Read the model definition and answer for the solid it produces. Units are mm, in the model's axes. A direction names the side the tool comes from. Give positions to 0.01 mm unless a question says otherwise; leave off trailing zeros. Loops run counter-clockwise (first coordinate to the right, second up) from the corner with the lowest first, then second, coordinate; pieces in that order, holes last. Notation, with made-up numbers: (-20, -18.5) -> (-14, -18.5) arc R26 ccw to (-14, -3.5) -> close; hole circle Ø8 at (19, 26). An arc over 180 degrees is marked (long way). Return JSON: item names as keys, results as strings. Group by question number.
from build123d import *

# Parameters (mm, degrees)
SALIENTE_EXTRUIR1_DEPTH                     = 31.75
CROQUIS1_R                                  = 9.525
CROQUIS1_R_2                                = 25.4
SALIENTE_EXTRUIR1_2_DEPTH                   = 31.75
SALIENTE_EXTRUIR2_DEPTH                     = 82.55
SALIENTE_EXTRUIR3_REACH                     = 71.85
TALADRO1_D                                  = 25.4
REFRENTADO_PARA_TORNILLO_CON_CABEZA_2_COUNT = 2
REFRENTADO_PARA_TORNILLO_CON_CABEZA_2_PITCH = 56.896
REFRENTADO_PARA_TORNILLO_CON_CABEZA_3_COUNT = 2
REFRENTADO_PARA_TORNILLO_CON_CABEZA_3_PITCH = 110.426919924


with BuildPart() as part:
    # Croquis1 → Saliente-Extruir1 (new body)
    with BuildSketch(Plane.XY):
        with BuildLine():
            Line((50.8, 170.942), (12.7, 170.942))
            Line((12.7, 170.942), (12.7, 154.94))
            Line((12.7, 154.94), (-12.7, 154.94))
            Line((-12.7, 154.94), (-12.7, 170.942))
            Line((-12.7, 170.942), (-50.8, 170.942))
            ThreePointArc((-50.8, 170.942), (-55.290128061, 169.082128061), (-57.15, 164.592))
            Line((-57.15, 164.592), (-57.15, 101.092))
            ThreePointArc((-57.15, 101.092), (-55.290128061, 105.582128061), (-50.8, 107.442))
            Line((-50.8, 107.442), (50.8, 107.442))
            ThreePointArc((50.8, 107.442), (55.290128061, 105.582128061), (57.15, 101.092))
            Line((57.15, 101.092), (57.15, 164.592))
            ThreePointArc((57.15, 164.592), (55.290128061, 169.082128061), (50.8, 170.942))
        make_face()
    extrude(amount=SALIENTE_EXTRUIR1_DEPTH)



with BuildPart() as body_2:
    # Croquis1 → Saliente-Extruir1 2 (new body)
    with BuildSketch(Plane.XY):
        with BuildLine():
            Line((57.15, 0), (57.15, 75.692))
            ThreePointArc((57.15, 75.692), (55.290128061, 71.201871939), (50.8, 69.342))
            Line((50.8, 69.342), (-50.8, 69.342))
            ThreePointArc((-50.8, 69.342), (-55.290128061, 71.201871939), (-57.15, 75.692))
            Line((-57.15, 75.692), (-57.15, 0))
            ThreePointArc((-57.15, 0), (0, -57.15), (57.15, 0))
        make_face()
        with Locations((0, -41.402)):
            Circle(CROQUIS1_R, mode=Mode.SUBTRACT)
        Circle(CROQUIS1_R_2, mode=Mode.SUBTRACT)
    extrude(amount=SALIENTE_EXTRUIR1_2_DEPTH)


with BuildPart() as part_1:
    add(part.part)

    add(body_2.part)  # Saliente-Extruir2 merges body 2
    # Croquis1_3 → Saliente-Extruir2 (add)
    with BuildSketch(Plane.XY):
        with BuildLine():
            Line((57.15, 75.692), (57.15, 101.092))
            ThreePointArc((57.15, 101.092), (55.290128061, 105.582128061), (50.8, 107.442))
            Line((50.8, 107.442), (-50.8, 107.442))
            ThreePointArc((-50.8, 107.442), (-55.290128061, 105.582128061), (-57.15, 101.092))
            Line((-57.15, 101.092), (-57.15, 75.692))
            ThreePointArc((-57.15, 75.692), (-55.290128061, 71.201871939), (-50.8, 69.342))
            Line((-50.8, 69.342), (50.8, 69.342))
            ThreePointArc((50.8, 69.342), (55.290128061, 71.201871939), (57.15, 75.692))
        make_face()
    extrude(amount=SALIENTE_EXTRUIR2_DEPTH)

    # Croquis4 → Saliente-Extruir3 (add, up to next)
    with BuildSketch(Plane.ZY.offset(-12.7), mode=Mode.PRIVATE) as saliente_extruir3_sk1:
        Polygon((31.75, 154.94), (0, 170.942), (0, 154.94), align=None)
    saliente_extruir3_tool1 = extrude(saliente_extruir3_sk1.sketch, amount=SALIENTE_EXTRUIR3_REACH, mode=Mode.PRIVATE) - part_1.part
    add(saliente_extruir3_tool1.solids().sort_by_distance((12.7, 160.274, 10.583333))[0])

    # Taladro1 (through all)
    with Locations(Plane(origin=(0, 107.442, 0), x_dir=(1, 0, 0), z_dir=(0, 1, 0))):
        with Locations((0, -57.15)):
            Hole(TALADRO1_D / 2)

    # Croquis10 → Refrentado para tornillo con cabeza tron (revolve, cut)
    with BuildSketch(Plane(origin=(28.448, 135.89, 31.75), x_dir=(0, -1, 0), z_dir=(1, 0, 0))):
        Polygon((0, 0), (0, 31.75), (6.35, 31.75), (6.35, 8.350483939), (6.985, 7.62), (8.001, 7.62), (8.001, 0), align=None)
    refrentado_para_tornillo_con_cabeza_tron = revolve(axis=Axis((28.448, 135.89, 38.1), (0, 0, -1)), mode=Mode.SUBTRACT)

    # Refrentado para tornillo con cabeza  2: Refrentado para tornillo con cabeza tron ×2
    with Locations(*[(-i * REFRENTADO_PARA_TORNILLO_CON_CABEZA_2_PITCH, 0, 0) for i in range(1, REFRENTADO_PARA_TORNILLO_CON_CABEZA_2_COUNT)]):
        add(refrentado_para_tornillo_con_cabeza_tron, mode=Mode.SUBTRACT)

    # Refrentado para tornillo con cabeza  3: Refrentado para tornillo con cabeza tron ×2
    with Locations(*[Vector(-0.517536847, -0.855660921, 0) * (i * REFRENTADO_PARA_TORNILLO_CON_CABEZA_3_PITCH) for i in range(1, REFRENTADO_PARA_TORNILLO_CON_CABEZA_3_COUNT)]):
        add(refrentado_para_tornillo_con_cabeza_tron, mode=Mode.SUBTRACT)


solid = part_1.part
1. Flat-ended cylindrical pins translate along their axes: pin 1 Ø5 at (y, z) = (49, 34) entering from +X; pin 2 Ø16.5 at (x, y) = (-28.448, 135.89) entering from +Z; pin 3 Ø1.5 at (x, z) = (45, 65) entering from -Y; pin 4 Ø9.5 at (x, y) = (28.448, 135.89) entering from -Z. Find the tip coordinate at first contact, or state that the pin passes through.
2. Straight lines are drawn through the part: line 1 (X direction, y = 135.89, z = 27); line 2 (X direction, y = 135.89, z = 18.25); line 3 (Z direction, x = 0, y = 79). For each, find the intervals that lie inside material, in ascending order. Write a range as from..to.
3. Section A-A on y = 135.89 is taken. Determine the outline of the cut face in (x, z).
4. Determine the mould class of faces 4 (the cylindrical face through (-55.34, 71.25, 56.79)), 5 (the cylindrical face through (-24.584, 140.929, 11.864)), 6 (the cylindrical face through (55.34, 169.03, 15.65)), 7 (the flat face through (12, 25, 31.75)) for opening direction X: pulls with the +X half, pulls with the -X half, needs draft (parallel to the pull), parting line crosses it, or undercut.
5. Section C-C on x = 0 is taken. Determine the outline of the cut face in (y, z).
6. Which of the six approach directions +Z, -Z, +X, -X, +Y, -Y give full straight-line access (tool end or side, diameter ignored) to faces 1 (the cylindrical face through (28.096, 143.883, 27.993)), 2 (the cylindrical face through (55.24, 71.15, 56.79)), 3 (the flat face through (12, 107.442, 51))?
7. Section D-D on z = 75.5 is taken. Determine the outline of the cut face in (x, y), then the cut area to 3 significant figures.
8. Section B-B on z = 57.15 is taken. Determine the outline of the cut face in (x, y).
Completed:
{
 "1": {"pin 1": "stops at x = 57.15", "pin 2": "stops at z = 31.75", "pin 3": "stops at y = 69.34", "pin 4": "passes through"},
 "2": {"line 1": "x = -57.15..-36.45, -20.45..20.45, 36.45..57.15", "line 2": "x = -57.15..-34.8, -22.1..22.1, 34.8..57.15", "line 3": "z = 0..44.45, 69.85..82.55"},
 "3": {"outline": "(-57.15, 0) -> (-34.8, 0) -> (-34.8, 23.4) -> (-35.43, 24.13) -> (-36.45, 24.13) -> (-36.45, 31.75) -> (-57.15, 31.75) -> close; (-22.1, 0) -> (22.1, 0) -> (22.1, 23.4) -> (21.46, 24.13) -> (20.45, 24.13) -> (20.45, 31.75) -> (-20.45, 31.75) -> (-20.45, 24.13) -> (-21.46, 24.13) -> (-22.1, 23.4) -> close; (34.8, 0) -> (57.15, 0) -> (57.15, 31.75) -> (36.45, 31.75) -> (36.45, 24.13) -> (35.43, 24.13) -> (34.8, 23.4) -> close"},
 "4": {"face 4": "pulls with the -X half", "face 5": "undercut", "face 6": "pulls with the +X half", "face 7": "needs draft"},
 "5": {"outline": "(-57.15, 0) -> (-50.93, 0) -> (-50.93, 31.75) -> (-57.15, 31.75) -> close; (-31.88, 0) -> (-25.4, 0) -> (-25.4, 31.75) -> (-31.88, 31.75) -> close; (25.4, 0) -> (170.94, 0) -> (154.94, 31.75) -> (107.44, 31.75) -> (107.44, 44.45) -> (69.34, 44.45) -> (69.34, 31.75) -> (25.4, 31.75) -> close; (69.34, 69.85) -> (107.44, 69.85) -> (107.44, 82.55) -> (69.34, 82.55) -> close"},
 "6": {"face 1": "+Z", "face 2": "+Z, +X, -Y", "face 3": "+Z, +X, -X, +Y"},
 "7": {"outline": "(-57.15, 75.69) arc R6.35 ccw to (-50.8, 69.34) -> (50.8, 69.34) arc R6.35 ccw to (57.15, 75.69) -> (57.15, 101.09) arc R6.35 ccw to (50.8, 107.44) -> (-50.8, 107.44) arc R6.35 ccw to (-57.15, 101.09) -> close", "area": "4,320 mm²"},
 "8": {"outline": "(-57.15, 75.69) arc R6.35 ccw to (-50.8, 69.34) -> (-12.7, 69.34) -> (-12.7, 107.44) -> (-50.8, 107.44) arc R6.35 ccw to (-57.15, 101.09) -> close; (12.7, 69.34) -> (50.8, 69.34) arc R6.35 ccw to (57.15, 75.69) -> (57.15, 101.09) arc R6.35 ccw to (50.8, 107.44) -> (12.7, 107.44) -> close"}
}
